```python
from build123d import *

# Parameters (mm, degrees)
BOSS_EXTRUDE5_DEPTH = 0.125
SKETCH1_W           = 1.5
SKETCH1_H           = 3
SKETCH1_W_2         = 4.66
SKETCH1_H_2         = 1.6
CUT_EXTRUDE2_DEPTH  = 62.727349085


with BuildPart() as part:
    # Sketch8 → Boss-Extrude5 (new body)
    with BuildSketch(Plane.XY):
        with BuildLine():
            Line((-12.5, 60), (4.5, 60))
            ThreePointArc((4.5, 60), (11.571067812, 57.071067812), (14.5, 50))
            Line((14.5, 50), (14.5, -58))
            ThreePointArc((14.5, -58), (13.914213562, -59.414213562), (12.5, -60))
            Line((12.5, -60), (-12.5, -60))
            ThreePointArc((-12.5, -60), (-13.914213562, -59.414213562), (-14.5, -58))
            Line((-14.5, -58), (-14.5, 58))
            ThreePointArc((-14.5, 58), (-13.914213562, 59.414213562), (-12.5, 60))
        make_face()
    extrude(amount=BOSS_EXTRUDE5_DEPTH)

    # Sketch1 → Cut-Extrude2 (cut, through all)
    with BuildSketch(Plane.XY.offset(0.125)):
        with BuildLine():
            Line((4.925, -48.85), (7.4, -46.97314145))
            add(Edge.make_bspline(
                [(7.4, -46.97314145), (8.211440188, -46.416320927), (8.75059415, -45.427724457), (8.75, -44.3)],
                knots=[3, 3, 3, 3, 3.998304655, 3.998304655, 3.998304655, 3.998304655], degree=3))
            add(Edge.make_bspline(
                [(8.75, -44.3), (8.749703343, -43.736930638), (8.614001568, -43.20601542), (8.375, -42.75)],
                knots=[2, 2, 2, 2, 3, 3, 3, 3], degree=3))
            Line((8.375, -42.75), (1.9, -29))
            Line((1.9, -29), (2.4, -29))
            Line((2.4, -29), (2.4, -6.15))
            Line((2.4, -6.15), (-2.4, -6.15))
            Line((-2.4, -6.15), (-2.4, -29))
            Line((-2.4, -29), (-1.9, -29))
            Line((-1.9, -29), (-8.375, -42.75))
            add(Edge.make_bspline(
                [(-8.375, -42.75), (-8.614001568, -43.20601542), (-8.749703343, -43.736930638), (-8.75, -44.3)],
                knots=[2, 2, 2, 2, 3, 3, 3, 3], degree=3))
            add(Edge.make_bspline(
                [(-8.75, -44.3), (-8.75059415, -45.427724457), (-8.211440188, -46.416320927), (-7.4, -46.97314145)],
                knots=[3, 3, 3, 3, 3.998304655, 3.998304655, 3.998304655, 3.998304655], degree=3))
            Line((-7.4, -46.97314145), (-4.925, -48.85))
            Line((-4.925, -48.85), (-2.6, -49.6))
            Line((-2.6, -49.6), (2.6, -49.6))
            Line((2.6, -49.6), (4.925, -48.85))
        make_face()
        with Locations((0, -52.1)):
            Rectangle(SKETCH1_W, SKETCH1_H)
        with Locations((6.41, -8.27)):
            Rectangle(SKETCH1_W_2, SKETCH1_H_2)
        with BuildLine():
            Line((-4, 16.031829774), (-4, 1.6))
            ThreePointArc((-4, 1.6), (-3.443502884, 0.256497116), (-2.1, -0.3))
            Line((-2.1, -0.3), (2.1, -0.3))
            ThreePointArc((2.1, -0.3), (3.443502884, 0.256497116), (4, 1.6))
            Line((4, 1.6), (4, 16.031829774))
            ThreePointArc((4, 16.031829774), (3.443502884, 17.375332658), (2.1, 17.931829774))
            Line((2.1, 17.931829774), (-2.1, 17.931829774))
            ThreePointArc((-2.1, 17.931829774), (-3.443502884, 17.375332658), (-4, 16.031829774))
        make_face()
        with BuildLine():
            Line((-4, 54.1), (-4, 38.9))
            ThreePointArc((-4, 38.9), (-3.443502884, 37.556497116), (-2.1, 37))
            Line((-2.1, 37), (2.1, 37))
            ThreePointArc((2.1, 37), (3.443502884, 37.556497116), (4, 38.9))
            Line((4, 38.9), (4, 54.1))
            ThreePointArc((4, 54.1), (3.443502884, 55.443502884), (2.1, 56))
            Line((2.1, 56), (-2.1, 56))
            ThreePointArc((-2.1, 56), (-3.443502884, 55.443502884), (-4, 54.1))
        make_face()
    extrude(amount=-CUT_EXTRUDE2_DEPTH, mode=Mode.SUBTRACT)


solid = part.part
```
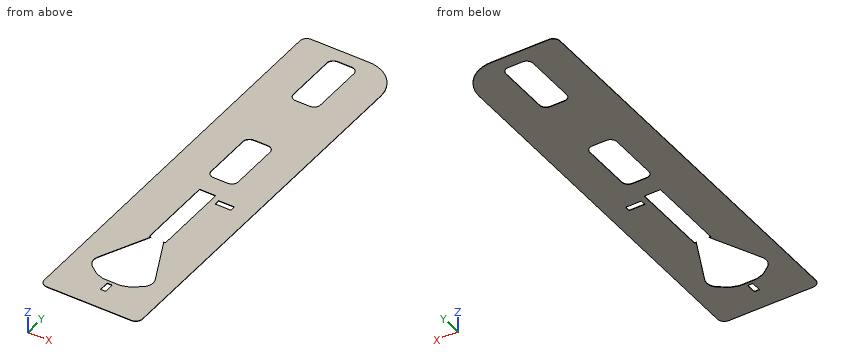
Input: part model. Units: mm. Frame: model coordinates. Round coordinates to 2 decimals unless told otherwise and drop trailing zeros. Loops run counter-clockwise (first coordinate to the right, second up) from the corner with the lowest first, then second, coordinate; pieces in that order, holes last. Notation, with made-up numbers: (46, 81.25) -> (54, 81.25) arc R20 cw to (54, 116.25) -> close; hole circle Ø11 at (64, 12.5). An arc over 180 degrees is marked (long way). Write each question's results on one line, items separated by ' | '.
1. First-contact query: P1, Ø6, axis at x = 1, y = 31.5, coming from the -Z side. Flat tip, straight axial feed; report the tip coordinate or a pass-through.
Geometry results:
P1: z = 0
2. Section B-B (y = -12). Return loops of the section in (x, z) (3 decimals).
Geometry results:
outline: (-14.5, 0) -> (-2.4, 0) -> (-2.4, 0.125) -> (-14.5, 0.125) -> close; (2.4, 0) -> (14.5, 0) -> (14.5, 0.125) -> (2.4, 0.125) -> close
3. Ray query, line 1 (Y direction, x = 6, z = 0.05); line 2 (Y direction, x = -3, z = 0.05); line 3 (X direction, y = -24, z = 0.05). Return the intervals inside material, ascending. Write a range as from..to.
Geometry results:
line 1: -60..-48.03, -37.71..-9.07, -7.47..59.89 | line 2: -60..-49.47, -31.34..-0.07, 17.71..37.23, 55.77..60 | line 3: -14.5..-2.4, 2.4..14.5
4. Section C-C (z = 0.05). State how many separate pieces and enclosed holes the cut face has, and give its area (3 significant figures).
Geometry results:
separate pieces: 1 | enclosed holes: 5 | area: 2,800 mm2
5. Section A-A (y = 7). Return loops of the section in (x, z) (3 decimals).
Geometry results:
outline: (-14.5, 0) -> (-4, 0) -> (-4, 0.125) -> (-14.5, 0.125) -> close; (4, 0) -> (14.5, 0) -> (14.5, 0.125) -> (4, 0.125) -> close
